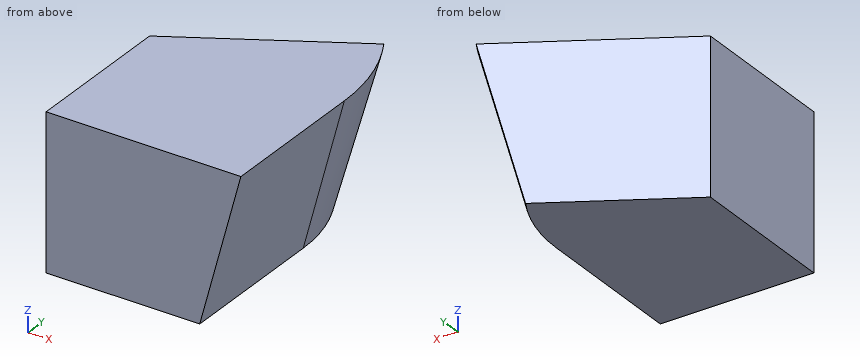
```python
from build123d import *

# Parameters (mm, degrees)
F1_DEPTH = 25.4
F2_ANGLE = 30


with BuildPart() as f1:
    # F0 (on Front) → F1 (new body)
    with BuildSketch(Plane.XZ):
        Polygon((0, 25.4), (0, 0), (25.4, 0), (32.205909, 25.4), align=None)
    extrude(amount=F1_DEPTH)

    # F0 (on Front) → F2 (revolve)
    with BuildSketch(Plane.XZ):
        Polygon((0, 25.4), (0, 0), (25.4, 0), (32.205909, 25.4), align=None)
    revolve(axis=Axis((0, 0, 12.7), (0, 0, 1)), revolution_arc=F2_ANGLE)


solid = f1.part
```
Geometry: final body of the model. Coordinates: model frame, mm. Coordinates: 2 decimals unless noted, no trailing zeros. Order: outer loops, then holes, each group sorted by start corner. A loop starts at its lowest first (then second) coordinate and runs counter-clockwise, first axis right, second up. Notation, with made-up numbers: (9.5, 88) - (22.5, 88) arc R16 cw to (22.5, 109) - close; hole circle Ø1 at (25, 19). An arc over 180 degrees is marked (long way). Return JSON: item names as keys, results as strings. Group by question number.
1. Material intervals for line 1 along Y through (x, z) = (11, 6.75); line 2 along Y through (x, z) = (8, 23.5); line 3 along X through (y, z) = (12, 10.5), sorted ascending. Write a range as [from, to].
2. Cut plane B-B (y = -19.5). Output: boundary loops of the cut face in (x, z).
3. Cut plane A-A (z = 2.75). Output: boundary loops of the cut face in (x, y), plus the area to 3 significant figures.
4. Pin query (flat end, axial travel): pin 1 (1 mm diameter, centred on x = 22.5, y = -9.5, fed in from -Z); pin 2 (1.5 mm diameter, centred on x = 20, z = 8, fed in from +Y); pin 3 (12 mm diameter, centred on y = -21, z = 11.5, fed in from +X); pin 4 (5 mm diameter, centred on x = 19, z = 20, fed in from +Y). Return the tip coordinate at first contact, or that it passes through.
5. Cut plane D-D (z = 17). Output: boundary loops of the cut face in (x, y).
6. Cut plane C-C (x = 18). Output: boundary loops of the cut face in (y, z), plus the area to 3 significant figures.
Resolved:
{
 "1": {"line 1": "y = [-25.4, 6.35]", "line 2": "y = [-25.4, 4.62]", "line 3": "x = [20.78, 25.53]"},
 "2": {"outline": "(0, 0) - (25.4, 0) - (32.21, 25.4) - (0, 25.4) - close"},
 "3": {"outline": "(0, -25.4) - (26.14, -25.4) - (26.14, 0) arc R26.14 ccw to (22.64, 13.07) - (0, 0) - close", "area": "843 mm²"},
 "4": {"pin 1": "stops at z = 0", "pin 2": "stops at y = 11.98", "pin 3": "stops at x = 30.09", "pin 4": "stops at y = 12.41"},
 "5": {"outline": "(0, -25.4) - (29.96, -25.4) - (29.96, 0) arc R29.96 ccw to (25.94, 14.98) - (0, 0) - close"},
 "6": {"outline": "(-25.4, 0) - (10.39, 0) - (10.39, 25.4) - (-25.4, 25.4) - close", "area": "909 mm²"}
}
